```python
from build123d import *

# Parameters (mm, degrees)
F3_D            = 12.7
F3_COPIES_COUNT = 6
F5_DEPTH        = 10.161
F5_COPIES_COUNT = 5
F5_COPIES_ANGLE = 240
F6_R            = 5.08
F7_SIZE         = 2.54


# Not quite as in the source:
# - a pattern or mirror of a feature is missing from the dataset's text; its kind, count and spacing are read off the source's solid


with BuildPart() as f1:
    # F0 (on Front) → F1 (revolve)
    with BuildSketch(Plane.XZ):
        Polygon((10.16, 0), (63.5, 0), (63.5, 10.16), (24.13, 10.16), (24.13, 20.6138496578), (10.16, 28.6794329184), align=None)
    revolve(axis=Axis((0, 0, 9.6584064886), (0, 0, 1)))

    # F3 (through all)
    with Locations(Plane.XY.offset(10.16)):
        with Locations((0, 50.8)):
            f3 = Hole(F3_D / 2)

    # F3_copies: F3 ×6 about axis
    f3_copies_axis = Axis((0, 0, 0), (0, 0, 1))
    for i in range(1, F3_COPIES_COUNT):
        add(f3.rotate(f3_copies_axis, i * 360 / F3_COPIES_COUNT), mode=Mode.SUBTRACT)

    # F4 (on face) → F5 (cut, through all)
    with BuildSketch(Plane.XY.offset(10.16)):
        with BuildLine():
            ThreePointArc((7.8888044947, 29.4414191853), (15.24, 26.3964543073), (21.5526146906, 21.5526146906))
            Line((21.5526146906, 21.5526146906), (40.4111525448, 40.4111525448))
            ThreePointArc((40.4111525448, 40.4111525448), (28.575, 49.4933518263), (14.7915084276, 55.2026609724))
            Line((14.7915084276, 55.2026609724), (7.8888044947, 29.4414191853))
        make_face()
    f5 = extrude(amount=-F5_DEPTH, mode=Mode.SUBTRACT)

    # F5_copies: F5 ×5 about axis
    f5_copies_axis = Axis((0, 0, 0), (0, 0, 1))
    for i in range(1, F5_COPIES_COUNT):
        add(f5.rotate(f5_copies_axis, i * F5_COPIES_ANGLE / (F5_COPIES_COUNT - 1)), mode=Mode.SUBTRACT)

    # F6
    f6_edges = [f1.edges().sort_by_distance(p)[0] for p in [
        (14.791508, 55.202661, 5.08),
        (7.888804, 29.441419, 5.08),
        (21.552615, 21.552615, 5.08),
        (40.411153, 40.411153, 5.08),
        (14.791508, -55.202661, 5.08),
        (7.888804, -29.441419, 5.08),
        (21.552615, -21.552615, 5.08),
        (40.411153, -40.411153, 5.08),
        (-40.411153, -40.411153, 5.08),
        (-21.552615, -21.552615, 5.08),
        (-14.791508, -55.202661, 5.08),
        (-7.888804, -29.441419, 5.08),
        (-55.202661, 14.791508, 5.08),
        (-29.441419, 7.888804, 5.08),
        (-55.202661, -14.791508, 5.08),
        (-29.441419, -7.888804, 5.08),
        (-14.791508, 55.202661, 5.08),
        (-7.888804, 29.441419, 5.08),
        (-40.411153, 40.411153, 5.08),
        (-21.552615, 21.552615, 5.08),
    ]]
    fillet(f6_edges, radius=F6_R)

    # F7
    f7_edges = [f1.edges().sort_by_distance(p)[0] for p in [
        (-63.5, 0, 10.16),
    ]]
    chamfer(f7_edges, length=F7_SIZE)


solid = f1.part
```
Work out the finished part from the listing and answer in its coordinate system (mm). A direction names the side the tool comes from. Coordinates: 2 decimals unless noted, no trailing zeros. Order: outer loops, then holes, each group sorted by start corner. A loop starts at its lowest first (then second) coordinate and runs counter-clockwise, first axis right, second up. Notation, with made-up numbers: (-6.75, 23) - (30.25, 23) arc R12 cw to (30.25, 39) - close; hole circle Ø6 at (53, 35). An arc over 180 degrees is marked (long way). Answer as a JSON object with one key per item and string values.
1. Find section C-C on y = 39. Count the separate pieces of the cut face and the enclosed holes in it, plus the area to 3 significant figures.
Output values:
{"separate pieces": "3", "enclosed holes": "0", "area": "451 mm²"}
2. The mould has two halves that part along X. Classify faces 3 (the face through (-42.14, -11.29, 5.15)), 4 (the face through (15.94, 53.23, 5.01)), 5 (the face through (1, -13, 0)), 6 (the face through (-1.411, 10.746, 28.288)): +X half, -X half, draft (parallel to the pull), parting line (faces both ways), or undercut.
Output values:
{"face 3": "undercut", "face 4": "undercut", "face 5": "draft", "face 6": "parting line"}
3. Find section B-B on z = 12.5. Determine the outline of the cut face in (x, y).
Output values:
{"outline": "circle Ø48.26 at (0, 0); hole circle Ø20.32 at (0, 0)"}
4. A tool of negligible diameter and unlimited length cuts with its end or side. For faces 1 (the face through (-31.076, -7.009, 5.009)), 2 (the face through (-48.47, -37.17, 10.04)), from which of +Z, -Z, +X, -X, +Y, -Y can it reach the whole face along a straight path? Write none if from no direction.
Output values:
{"face 1": "+Z, -Z", "face 2": "+Z"}
5. Find section D-D on z = 23.25. Determine the outline of the cut face in (x, y), plus the area to 3 significant figures.
Output values:
{"outline": "circle Ø39.13 at (0, 0); hole circle Ø20.32 at (0, 0)", "area": "878 mm²"}
6. Each of these flat-tipped pins is pushed along its axis until it touches: P1, Ø12, axis at x = 13.5, z = 6.5, coming from the -Y side; P2, Ø2, axis at x = -43, z = 9, coming from the +Y side; P3, Ø20.5, axis at x = 0, y = 50.8, coming from the +Z side; P4, Ø2, axis at y = 34, z = 11.5, coming from the -X side. Where does it stop, or does it pass through?
Output values:
{"P1": "stops at y = -63.06", "P2": "stops at y = 46.49", "P3": "stops at z = 10.16", "P4": "passes through"}
7. Consider line 1 (Y direction, x = 0, z = 7); line 2 (Y direction, x = -28.5, z = 7.5); line 3 (Y direction, x = 29, z = 2.5). Determine where each line is inside the solid, lowest interval first.
Output values:
{"line 1": "y = -63.5 to -57.15, -44.45 to -10.16, 10.16 to 44.45, 57.15 to 63.5", "line 2": "y = -56.75 to -49.54, -28.5 to 28.5, 49.54 to 56.75", "line 3": "y = -56.49 to -49.25, -29 to 29, 49.25 to 56.49"}
8. Find section A-A on x = 0. Determine the outline of the cut face in (y, z), plus the area to 3 significant figures.
Output values:
{"outline": "(-63.5, 0) - (-57.15, 0) - (-57.15, 10.16) - (-60.96, 10.16) - (-63.5, 7.62) - close; (-44.45, 0) - (-10.16, 0) - (-10.16, 28.68) - (-24.13, 20.61) - (-24.13, 10.16) - (-44.45, 10.16) - close; (10.16, 0) - (44.45, 0) - (44.45, 10.16) - (24.13, 10.16) - (24.13, 20.61) - (10.16, 28.68) - close; (57.15, 0) - (63.5, 0) - (63.5, 7.62) - (60.96, 10.16) - (57.15, 10.16) - close", "area": "1,220 mm²"}
